Autodesk Inventor part; units mm, degrees
ref_plane "YZ Plane" through (0, 0, 0) normal (1, 0, 0) x (0, 1, 0)
ref_plane "XZ Plane" through (0, 0, 0) normal (0, 1, 0) x (-1, 0, 0)
ref_plane "XY Plane" through (0, 0, 0) normal (0, 0, 1) x (1, 0, 0)
sketch "Sketch1" plane through (0, 0, 0) normal (0, 0, 1) x (1, 0, 0)
  circle A0 centre (0, 0) radius 2.4 construction
  line L0 (-0.8, 2.2627) -> (-0.8, 0.8)
  line L1 (-0.8, 0.8) -> (-2.2627, 0.8)
  line L2 (-2.2627, -0.8) -> (-0.8, -0.8)
  line L3 (-0.8, -0.8) -> (-0.8, -2.2627)
  line L4 (0.8, -2.2627) -> (0.8, -0.8)
  line L5 (0.8, -0.8) -> (2.2627, -0.8)
  line L6 (2.2627, 0.8) -> (0.8, 0.8)
  line L7 (0.8, 0.8) -> (0.8, 2.2627)
  arc A1 (0.8, 2.2627) -> (-0.8, 2.2627) centre (0, 0) ccw
  arc A2 (-2.2627, 0.8) -> (-2.2627, -0.8) centre (0, 0) ccw
  arc A3 (-0.8, -2.2627) -> (0.8, -2.2627) centre (0, 0) ccw
  arc A4 (2.2627, -0.8) -> (2.2627, 0.8) centre (0, 0) ccw
  dimension "d0" = 4.8
  dimension "d1" = 1.6
extrude "Extrusion1" add sketch "Sketch1" along normal mid plane 16
fillet "Fillet1" radius 0.4 8 edges at (0, 2.4, 8) (-2.4, 0, 8) (0, -2.4, 8) (2.4, 0, 8) (2.4, 0, -8) (0, 2.4, -8) (-2.4, 0, -8) (0, -2.4, -8)
sketch "Sketch2" plane through (0, 0, 0) normal (1, 0, 0) x (0, 1, 0)
  line L0 (-2.4, -7.6) -> (-2.4, 7.6)
  line L1 (0, -10.64) -> (0, 10.64)
  line L2 (-2.4, 4.5) -> (-1.4, 4.5)
  line L3 (-1.4, 4.5) -> (-1.4, 3.5)
  line L4 (-1.4, 3.5) -> (-2.4, 3.5)
  line L5 (-2.4, 3.5) -> (-2.4, 4.5)
  line L6 (-2.4, -4.5) -> (-1.4, -4.5)
  line L7 (-1.4, -4.5) -> (-1.4, -3.5)
  line L8 (-1.4, -3.5) -> (-2.4, -3.5)
  line L9 (-2.4, -3.5) -> (-2.4, -4.5)
  line L10 (-1.4, 3.5) -> (-1.4, -3.5) construction
  point P0 (0, 0)
  point P1 (-2.4, 4)
  point P2 (-2.4, -4)
  point P3 (-1.4, 0)
  dimension "d7" = 8
  dimension "d8" = 1
revolve "Revolution1" cut sketch "Sketch2" angle 360 about axis through (0, 0, -10) along (0, 0, 1)
equation "\"d0\" = kd"
equation "\"d1\" = axlet"
equation "\"d2\" = 2 * lu"
equation "\"d4\" = tf"
properties part number "32062-Red" material "ABS Plastic"
Can you work these out from the model? Positions are in its coordinate system, mm. A direction names the side the tool comes from. Round coordinates to 2 decimals unless told otherwise and drop trailing zeros. Order: outer loops, then holes, each group sorted by start corner. A loop starts at its lowest first (then second) coordinate and runs counter-clockwise, first axis right, second up. Notation, with made-up numbers: M -37.5,69.25 L 12.5,69.25 A21 cw 12.5,108.25 Z; hole C 28.5,57 d1. An arc over 180 degrees is marked long. Use a Markdown table: item, result.
1) I'm going to push flat-ended pins straight in: P1, Ø0.6, axis at x = 0.5, y = -2, coming from the -Z side; P2, Ø0.7, axis at y = 1.5, z = -1.5, coming from the +X side; P3, Ø0.7, axis at y = 1.5, z = 3.5, coming from the -X side; P4, Ø1.2, axis at x = -1.5, z = 0, coming from the -Y side. Where does each tip first touch, or does it pass through?
Geometry says:
| item | result |
|---|---|
| P1 | stops at z = -8 |
| P2 | stops at x = 0.8 |
| P3 | stops at x = -0.8 |
| P4 | stops at y = -0.8 |
2) If we mould it in two halves opening along Z, with no side actions, what happens to faces 4 (the face through (0, 0, -8)), 5 (the face through (1.4, 0, -4)), 6 (the face through (0, 2, -3.5)), 7 (the face through (2, -0.8, 0))? For each: +Z half, -Z half, draft (parallel to the pull), parting line (faces both ways), or undercut.
Geometry says:
| item | result |
|---|---|
| face 4 | -Z half |
| face 5 | undercut |
| face 6 | undercut |
| face 7 | draft |
3) Imagine slicing it at A-A (z = 4.25). List the corners of the cut face in (x, y) for me, then the cut area to 3 significant figures.
Geometry says:
| item | result |
|---|---|
| outline | M -1.15,-0.8 L -0.8,-0.8 L -0.8,-1.15 A1.4 ccw 0.8,-1.15 L 0.8,-0.8 L 1.15,-0.8 A1.4 ccw 1.15,0.8 L 0.8,0.8 L 0.8,1.15 A1.4 ccw -0.8,1.15 L -0.8,0.8 L -1.15,0.8 A1.4 ccw Z |
| area | 5.89 mm² |
4) On a 3-axis mill with a long thin cutter (end or side, diameter ignored), from which of +Z, -Z, +X, -X, +Y, -Y can I reach the whole of each face in a straight line? I mean faces 1 (the face through (0, 1.4, -4)), 2 (the face through (0.8, -2, 0)), 3 (the face through (0, -1.4, 4)). Say none if no direction works.
Geometry says:
| item | result |
|---|---|
| face 1 | +Y |
| face 2 | +Z, -Z, +X, -Y |
| face 3 | -Y |
5) Imagine slicing it at B-B (x = -0.95). List the corners of the cut face in (y, z) for me, then the cut area to 3 significant figures.
Geometry says:
| item | result |
|---|---|
| outline | M -0.8,-8 L 0.8,-8 L 0.8,8 L -0.8,8 Z |
| area | 25.6 mm² |
6) If I drill on line 1 along Y through (x, z) = (-1.95, -6); line 2 along X through (y, z) = (-0.1, -4), over which ranges is the centre line in solid material (lowest first)?
Geometry says:
| item | result |
|---|---|
| line 1 | y = -0.8 to 0.8 |
| line 2 | x = -1.4 to 1.4 |
